```python
from build123d import *

# Parameters (mm, degrees)
SKETCH1_W               = 7.8
SKETCH1_H               = 10.9
BOSS_EXTRUDE1_DEPTH     = 20
SKETCH2_W               = 11.9
SKETCH2_H               = 15
BOSS_EXTRUDE2_DEPTH     = 50
CUT_EXTRUDE1_DEPTH      = 72.399299716
CUT_EXTRUDE1_DEPTH_BACK = 72.399299716
FILLET1_R               = 3


with BuildPart() as part:
    # Sketch1 → Boss-Extrude1 (new body)
    with BuildSketch(Plane(origin=(0, 0, 0), x_dir=(1, 0, 0), z_dir=(0, 1, 0))):
        Rectangle(SKETCH1_W, SKETCH1_H)
    extrude(amount=BOSS_EXTRUDE1_DEPTH)

    # Sketch2 → Boss-Extrude2 (add)
    with BuildSketch(Plane(origin=(0, 20, 0), x_dir=(1, 0, 0), z_dir=(0, 1, 0))):
        Rectangle(SKETCH2_W, SKETCH2_H)
    extrude(amount=BOSS_EXTRUDE2_DEPTH)

    # Sketch3 → Cut-Extrude1 (cut, two sides: drawn at the far end of the back side and taken through both)
    with BuildSketch(Plane.ZY.offset(5.95).offset(-CUT_EXTRUDE1_DEPTH_BACK)):
        Polygon((-7.5, 20), (-1.5, 70), (-7.5, 70), align=None)
    extrude(amount=CUT_EXTRUDE1_DEPTH + CUT_EXTRUDE1_DEPTH_BACK, mode=Mode.SUBTRACT)

    # Fillet1
    fillet1_edges = [part.edges().sort_by_distance(p)[0] for p in [
        (5.95, 45, 7.5),
        (-5.95, 45, 7.5),
    ]]
    fillet(fillet1_edges, radius=FILLET1_R)


solid = part.part
```
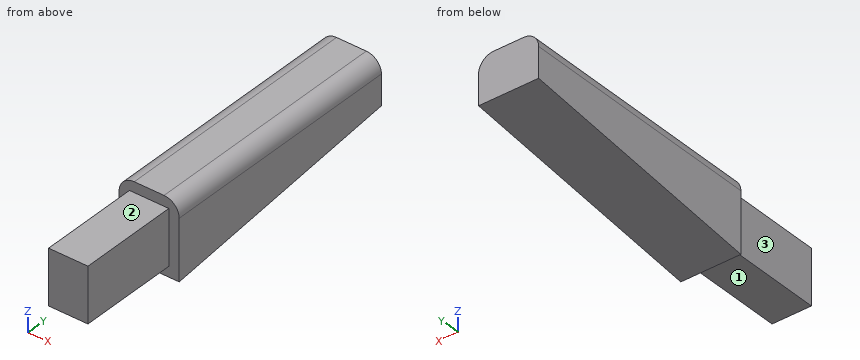
Build history of the part. All positions in model axes, mm. Face numbers are marked on the shaded views. A direction names the side the tool comes from. Give positions to 0.01 mm unless a question says otherwise; leave off trailing zeros. Loops run counter-clockwise (first coordinate to the right, second up) from the corner with the lowest first, then second, coordinate; pieces in that order, holes last. Notation, with made-up numbers: (3, 28.5) - (20, 28.5) arc R29 cw to (20, 55.5) - close; hole circle Ø11 at (17.25, 18.25). An arc over 180 degrees is marked (long way). Use a Markdown table: item, result.
(1) Which spindle directions (+Z, -Z, +X, -X, +Y, -Y) get a long thin tool onto all of the face, cutting with end or side? Do the marked faces 1, 2 and 3. Say none if no direction does.
Taken from the geometry:
| item | result |
|---|---|
| face 1 | -Z, +X, -X, -Y |
| face 2 | +Z, +X, -X, -Y |
| face 3 | +Z, -Z, -X, -Y |
(2) Band-saw the part on A-A (x = 0.5). Give the cut face in (y, z).
Taken from the geometry:
| item | result |
|---|---|
| outline | (0, -5.45) - (20, -5.45) - (20, -7.5) - (70, -1.5) - (70, 7.5) - (20, 7.5) - (20, 5.45) - (0, 5.45) - close |
(3) Band-saw the part on B-B (z = 0.25). Give the cut face in (x, y), and give its area (3 significant figures).
Taken from the geometry:
| item | result |
|---|---|
| outline | (-5.95, 20) - (-3.9, 20) - (-3.9, 0) - (3.9, 0) - (3.9, 20) - (5.95, 20) - (5.95, 70) - (-5.95, 70) - close |
| area | 751 mm2 |
(4) Drop flat-ended pins along their axis: pin 1 Ø5 at (x, z) = (1.5, -1) entering from -Y; pin 2 Ø1.5 at (y, z) = (7.5, -1) entering from -X; pin 3 Ø1.5 at (x, y) = (-3, 43) entering from -Z; pin 4 Ø5.5 at (y, z) = (14.5, 2.5) entering from +X. Give the stop position or say it passes through.
Taken from the geometry:
| item | result |
|---|---|
| pin 1 | y = 0 |
| pin 2 | x = -3.9 |
| pin 3 | z = -4.83 |
| pin 4 | x = 3.9 |
(5) Band-saw the part on D-D (y = 58). Give the cut face in (x, z).
Taken from the geometry:
| item | result |
|---|---|
| outline | (-5.95, -2.94) - (5.95, -2.94) - (5.95, 4.5) arc R3 ccw to (2.95, 7.5) - (-2.95, 7.5) arc R3 ccw to (-5.95, 4.5) - close |
(6) Band-saw the part on C-C (y = 21.5). Give the cut face in (x, z).
Taken from the geometry:
| item | result |
|---|---|
| outline | (-5.95, -7.32) - (5.95, -7.32) - (5.95, 4.5) arc R3 ccw to (2.95, 7.5) - (-2.95, 7.5) arc R3 ccw to (-5.95, 4.5) - close |
(7) Wall check: line 1 along Z through (x, y) = (0.25, 17); line 2 along Y through (x, z) = (-5, 4.75); line 3 along X through (y, z) = (3, -0.5). Give the ranges that are in metal, low to high.
Taken from the geometry:
| item | result |
|---|---|
| line 1 | -5.45 to 5.45 |
| line 2 | 20 to 70 |
| line 3 | -3.9 to 3.9 |
